Geometry: final body of the model. Coordinates: model frame, mm. Face numbers are marked on the shaded views. A direction names the side the tool comes from. Coordinates: 2 decimals unless noted, no trailing zeros. Loops run counter-clockwise (first coordinate to the right, second up) from the corner with the lowest first, then second, coordinate; pieces in that order, holes last. Notation, with made-up numbers: M 48.25,52.25 L 94.25,52.25 A16 ccw 94.25,64.25 Z; hole C -26,-14 d11. An arc over 180 degrees is marked long. Write each question's results on one line, items separated by ' | '. Start each with the question number.
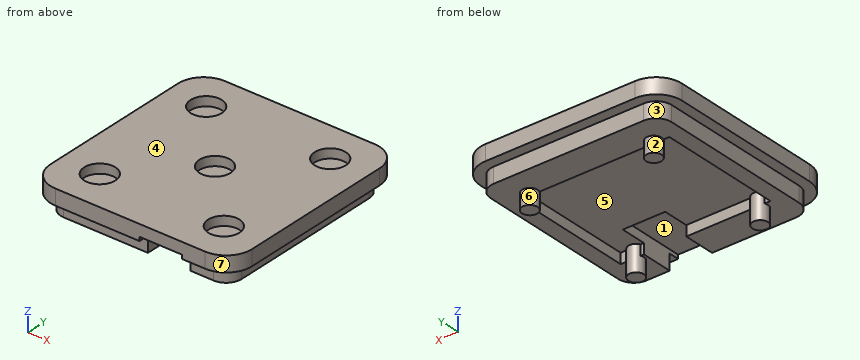
Autodesk Fusion 360 part; units mm, degrees
sketch "Outline camera" plane through (0, 0, 0) normal (0, 0, 1) x (1, 0, 0)
  line L0 (-6.5, 6.5) -> (-2.5981, 6.5)
  line L1 (2.5981, 6.5) -> (6.5, 6.5)
  arc A0 (6.7082, 2) -> (6.5, 2.5981) centre (0, 0) ccw
  arc A1 (2.5981, 6.5) -> (-2.5981, 6.5) centre (0, 0) ccw
  line L2 (6.7082, 2) -> (9, 2)
  line L3 (6.5, 6.5) -> (6.5, 2.5981)
  line L4 (6.5, -2.5981) -> (6.5, -6.5)
  arc A2 (9, -2) -> (9, 2) centre (9, 0) ccw
  line L5 (9, -2) -> (6.7082, -2)
  arc A3 (6.5, -2.5981) -> (6.7082, -2) centre (0, 0) ccw
  line L6 (6.5, -6.5) -> (2.5981, -6.5)
  line L7 (-2.5981, -6.5) -> (-6.5, -6.5)
  line L8 (-9, 2) -> (-6.7082, 2)
  line L9 (-6.7082, -2) -> (-9, -2)
  line L10 (-6.5, -6.5) -> (-6.5, -2.5981)
  line L11 (-6.5, 2.5981) -> (-6.5, 6.5)
  arc A4 (-9, 2) -> (-9, -2) centre (-9, 0) ccw
  arc A5 (-6.5, 2.5981) -> (-6.7082, 2) centre (0, 0) ccw
  arc A6 (-6.7082, -2) -> (-6.5, -2.5981) centre (0, 0) ccw
  arc A7 (-2.5981, -6.5) -> (2.5981, -6.5) centre (0, 0) ccw
  arc A8 (2.6926, 7) -> (-2.6926, 7) centre (0, 0) ccw
  line L12 (-7, 7) -> (-2.6926, 7)
  line L13 (-7, 2.6926) -> (-7, 7)
  arc A9 (-7, 2.6926) -> (-7.0711, 2.5) centre (0, 0) ccw
  line L14 (-9, 2.5) -> (-7.0711, 2.5)
  arc A10 (-9, 2.5) -> (-9, -2.5) centre (-9, 0) ccw
  line L15 (-7.0711, -2.5) -> (-9, -2.5)
  arc A11 (-7.0711, -2.5) -> (-7, -2.6926) centre (0, 0) ccw
  line L16 (-7, -7) -> (-7, -2.6926)
  line L17 (-2.6926, -7) -> (-7, -7)
  arc A12 (-2.6926, -7) -> (2.6926, -7) centre (0, 0) ccw
  line L18 (7, -7) -> (2.6926, -7)
  line L19 (7, -2.6926) -> (7, -7)
  arc A13 (7, -2.6926) -> (7.0711, -2.5) centre (0, 0) ccw
  line L20 (9, -2.5) -> (7.0711, -2.5)
  arc A14 (9, -2.5) -> (9, 2.5) centre (9, 0) ccw
  line L21 (7.0711, 2.5) -> (9, 2.5)
  arc A15 (7.0711, 2.5) -> (7, 2.6926) centre (0, 0) ccw
  line L22 (7, 7) -> (7, 2.6926)
  line L23 (2.6926, 7) -> (7, 7)
  dimension "d3" = 13
  dimension "d4" = 13
  dimension "d5" = 14
  dimension "d6" = 4
  dimension "d7" = 4
  dimension "d8" = 2
  dimension "d9" = 2
  dimension "d11" = 9
  dimension "d12" = 9
  dimension "d18" = -0.5
sketch "Box size" plane through (0, 0, 0) normal (0, 0, 1) x (1, 0, 0)
  line L0 (19.5, 20.125) -> (-19.5, 20.125)
  line L1 (-19.5, 20.125) -> (-19.5, -20.125)
  line L2 (-19.5, -20.125) -> (19.5, -20.125)
  line L3 (19.5, -20.125) -> (19.5, 20.125)
  line L4 (19.5, 20.125) -> (-19.5, -20.125) construction
  line L5 (-19.5, 20.125) -> (19.5, -20.125) construction
  line L6 (-14.5, -18.125) -> (14.5, -18.125)
  line L7 (17.5, -15.125) -> (17.5, 15.125)
  line L8 (14.5, 18.125) -> (-14.5, 18.125)
  line L9 (-17.5, 15.125) -> (-17.5, -15.125)
  arc A0 (17.5, 15.125) -> (14.5, 18.125) centre (14.5, 15.125) ccw
  arc A1 (-14.5, 18.125) -> (-17.5, 15.125) centre (-14.5, 15.125) ccw
  arc A2 (14.5, -18.125) -> (17.5, -15.125) centre (14.5, -15.125) ccw
  arc A3 (-17.5, -15.125) -> (-14.5, -18.125) centre (-14.5, -15.125) ccw
  dimension "d13" = 39
  dimension "d14" = 40.25
  dimension "d47" = 3
sketch "LEDs" plane through (0, 0, 0) normal (0, 0, 1) x (1, 0, 0)
  circle A0 centre (-12.5, 6) radius 2.4
  line L0 (0, 2.5) -> (0, 20)
  circle A1 centre (12.5, 6) radius 2.4
  line L1 (20, 0) -> (2.5, 0)
  circle A2 centre (-12.5, -6) radius 2.4
  circle A3 centre (12.5, -6) radius 2.4
  dimension "d15" = 4.8
  dimension "d16" = 12.5
  dimension "d17" = 6
extrude "Extrude1" add sketch "Box size" along normal blind 6 contours L0 L1 L2 L3 | L6 L7 L8 L9 A0 A1 A2 A3
sketch "Pins" plane through (0, 0, 0) normal (0, 0, 1) x (1, 0, 0)
  line L0 (12, 12.625) -> (-12, 12.625)
  line L1 (-12, 12.625) -> (-12, -12.625)
  line L2 (-12, -12.625) -> (12, -12.625)
  line L3 (12, -12.625) -> (12, 12.625)
  line L4 (12, 12.625) -> (-12, -12.625) construction
  line L5 (-12, 12.625) -> (12, -12.625) construction
  circle A0 centre (-12, -12.625) radius 1.5
  circle A1 centre (12, -12.625) radius 1.5
  circle A2 centre (12, 12.625) radius 1.5
  circle A3 centre (-12, 12.625) radius 1.5
  dimension "d35" = 24
  dimension "d36" = 25.25
  dimension "d37" = 3
extrude "Extrude4" add sketch "Pins" against normal blind 3 contours L0 L1 A3 | L0 L1 A3 | L0 L3 A2 | L0 L3 A2 | L1 L2 A0 | L1 L2 A0 | L2 L3 A1 | L2 L3 A1
fillet "Fillet2" radius 5 4 edges at (-19.5, 20.125, 3) (-19.5, -20.125, 3) (19.5, -20.125, 3) (19.5, 20.125, 3)
extrude "Extrude6" cut sketch "Box size" along normal blind 3
sketch "Sketch15" plane through (0, 0, 0) normal (0, 0, -1) x (1, 0, 0)
  circle A0 centre (-12, -12.625) radius 1.5
  circle A1 centre (-12, 12.625) radius 1.5
  circle A2 centre (12, -12.625) radius 1.5
  circle A3 centre (12, 12.625) radius 1.5
  arc A4 (-14.5, 18.125) -> (-17.5, 15.125) centre (-14.5, 15.125) ccw
  line L0 (-17.5, 15.125) -> (-17.5, -15.125)
  arc A5 (-17.5, -15.125) -> (-14.5, -18.125) centre (-14.5, -15.125) ccw
  line L1 (-14.5, -18.125) -> (14.5, -18.125)
  arc A6 (14.5, -18.125) -> (17.5, -15.125) centre (14.5, -15.125) ccw
  line L2 (17.5, -15.125) -> (17.5, 15.125)
  arc A7 (17.5, 15.125) -> (14.5, 18.125) centre (14.5, 15.125) ccw
  line L3 (14.5, 18.125) -> (-14.5, 18.125)
  line L4 (-14.5, 12) -> (14.5, 12)
  line L5 (14.5, 12) -> (14.5, -12)
  line L6 (14.5, -12) -> (-14.5, -12)
  line L7 (-14.5, -12) -> (-14.5, 12)
  line L8 (-14.5, 12) -> (14.5, -12) construction
  line L9 (14.5, 12) -> (-14.5, -12) construction
  dimension "d55" = 29
  dimension "d56" = 24
extrude "Extrude11" cut sketch "Sketch15" against normal blind 2 contours A0 A1 A2 A3 L4 L5 L6 L7
sketch "cable" plane through (0, 0, 0) normal (0, 0, -1) x (1, 0, 0)
  line L0 (-14.5, -12) -> (-13.3636, -12)
  arc A0 (-10.6364, -12) -> (-13.3636, -12) centre (-12, -12.625) ccw
  line L1 (-10.6364, -12) -> (10.6364, -12)
  arc A1 (13.3636, -12) -> (10.6364, -12) centre (12, -12.625) ccw
  line L2 (13.3636, -12) -> (14.5, -12)
  line L3 (14.5, -12) -> (14.5, 12)
  line L4 (14.5, 12) -> (13.3636, 12)
  arc A2 (10.6364, 12) -> (13.3636, 12) centre (12, 12.625) ccw
  line L5 (10.6364, 12) -> (-10.6364, 12)
  arc A3 (-13.3636, 12) -> (-10.6364, 12) centre (-12, 12.625) ccw
  line L6 (-13.3636, 12) -> (-14.5, 12)
  line L7 (-14.5, 12) -> (-14.5, -12)
  line L8 (10, 7) -> (1.8, 7)
  line L9 (1.8, 7) -> (1.8, 27)
  line L10 (1.8, 27) -> (10, 27)
  line L11 (10, 27) -> (10, 7)
  line L12 (14.5, 18.125) -> (-14.5, 18.125)
  arc A4 (-14.5, 18.125) -> (-17.5, 15.125) centre (-14.5, 15.125) ccw
  line L13 (-17.5, 15.125) -> (-17.5, -15.125)
  arc A5 (-17.5, -15.125) -> (-14.5, -18.125) centre (-14.5, -15.125) ccw
  line L14 (-14.5, -18.125) -> (14.5, -18.125)
  arc A6 (14.5, -18.125) -> (17.5, -15.125) centre (14.5, -15.125) ccw
  line L15 (17.5, -15.125) -> (17.5, 15.125)
  arc A7 (17.5, 15.125) -> (14.5, 18.125) centre (14.5, 15.125) ccw
  line L16 (13.3636, 12) -> (14.5, 12)
  line L17 (14.5, 12) -> (14.5, -12)
  line L18 (14.5, -12) -> (13.3636, -12)
  arc A8 (10.6364, -12) -> (13.3636, -12) centre (12, -12.625) ccw
  line L19 (10.6364, -12) -> (-10.6364, -12)
  arc A9 (-13.3636, -12) -> (-10.6364, -12) centre (-12, -12.625) ccw
  line L20 (-13.3636, -12) -> (-14.5, -12)
  line L21 (-14.5, -12) -> (-14.5, 12)
  line L22 (-14.5, 12) -> (-13.3636, 12)
  arc A10 (-10.6364, 12) -> (-13.3636, 12) centre (-12, 12.625) ccw
  line L23 (-10.6364, 12) -> (10.6364, 12)
  arc A11 (13.3636, 12) -> (10.6364, 12) centre (12, 12.625) ccw
  dimension "d67" = 8.2
  dimension "d68" = 2
  dimension "d69" = 20
extrude "Extrude12" cut sketch "cable" against normal blind 3.75 contours L5 L9 L11 L12 L23 | L5 L8 L9 L11 L23 | L9 L10 L11 L12
sketch "Sketch17" plane through (0, 0, 6) normal (0, 0, 1) x (-1, 0, 0)
  arc A0 (-19.5, -15.125) -> (-14.5, -20.125) centre (-14.5, -15.125) ccw
  line L0 (-14.5, -20.125) -> (14.5, -20.125)
  arc A1 (14.5, -20.125) -> (19.5, -15.125) centre (14.5, -15.125) ccw
  line L1 (19.5, -15.125) -> (19.5, 15.125)
  arc A2 (19.5, 15.125) -> (14.5, 20.125) centre (14.5, 15.125) ccw
  line L2 (14.5, 20.125) -> (-14.5, 20.125)
  arc A3 (-14.5, 20.125) -> (-19.5, 15.125) centre (-14.5, 15.125) ccw
  line L3 (-19.5, 15.125) -> (-19.5, -15.125)
  circle A4 centre (-12, 12.625) radius 3.025
  circle A5 centre (0, 0) radius 3.025
  dimension "d72" = 6.05
  dimension "d75" = 7.5
  dimension "d76" = 7.5
extrude "Extrude13" cut sketch "Sketch17" against normal blind 1.8 contours A4 | A5
mirror "Mirror1" about plane through (0, 0, 0) normal (0, 1, 0) of "Extrude13"
mirror "Mirror2" about plane through (0, 0, 0) normal (1, 0, 0) of "Extrude13", "Mirror1"
equation "d13 = 34 mm + 5 mm"
equation "d14 = 32 mm + 4 mm - 1 mm + 0.25 mm + 5 mm"
equation "d36 = 22 mm + 4 mm - 1 mm + 0.25 mm"
Item 1: Section A-A, the plane y = 0. Return loops of the section in (x, z) (3 decimals).
Item 2: Pull-direction query (Y, two-part tool) for the marked faces 4, 5, 6 and 7; classes: released by +Y, released by -Y, zero draft, split by the parting line, or undercut.
Item 3: Section D-D, the plane x = 0. Return loops of the section in (y, z) (3 decimals).
Item 4: Contact query for flat-ended pins moving along their axis: P1, Ø1, axis at x = 1, z = 1.5, coming from the -Y side (3 decimals); P2, Ø3, axis at x = -10.5, y = -2.5, coming from the -Z side; P3, Ø0.9, axis at x = 6, z = 1, coming from the +Y side (3 decimals). Output: stop coordinate, or through.
Item 5: Section C-C, the plane z = 0.5. Return loops of the section in (x, y) (3 decimals), plus the area to 3 significant figures.
Item 6: Section B-B, the plane x = -12. Return loops of the section in (y, z) (3 decimals), plus the area to 3 significant figures.
Item 7: Set-up query: the marked faces 1, 2 and 3. Return all of +Z, -Z, +X, -X, +Y, -Y with unobstructed straight access to the full face (end or side cutting, diameter ignored); none if empty.
Item 8: Ray query, L1, parallel to Y at x = -12, z = 4.95 (3 decimals); L2, parallel to X at y = 10, z = 4.25; L3, parallel to Y at x = 0, z = 4.9 (3 decimals). Return the intervals inside material, ascending. Write a range as [from, to].
Solutions:
1) outline: M -19.5,3 L -17.5,3 L -17.5,0 L -14.5,0 L -14.5,2 L 14.5,2 L 14.5,0 L 17.5,0 L 17.5,3 L 19.5,3 L 19.5,6 L 3.025,6 L 3.025,4.2 L -3.025,4.2 L -3.025,6 L -19.5,6 Z
2) face 4: zero draft | face 5: undercut | face 6: undercut | face 7: released by -Y
3) outline: M -20.125,3 L -18.125,3 L -18.125,0 L -12,0 L -12,2 L 12,2 L 12,0 L 18.125,0 L 18.125,3 L 20.125,3 L 20.125,6 L 3.025,6 L 3.025,4.2 L -3.025,4.2 L -3.025,6 L -20.125,6 Z
4) P1: stops at y = -18.125 | P2: stops at z = 2 | P3: stops at y = 18.125
5) outline: M -17.5,-15.125 A3 ccw -14.5,-18.125 L 1.8,-18.125 L 1.8,-12 L -10.636,-12 A1.5 ccw -13.364,-12 L -14.5,-12 L -14.5,12 L -13.364,12 A1.5 ccw -10.636,12 L 10.636,12 A1.5 ccw 13.364,12 L 14.5,12 L 14.5,-12 L 13.364,-12 A1.5 ccw 10.636,-12 L 10,-12 L 10,-18.125 L 14.5,-18.125 A3 ccw 17.5,-15.125 L 17.5,15.125 A3 ccw 14.5,18.125 L -14.5,18.125 A3 ccw -17.5,15.125 Z | area: 522 mm²
6) outline: M -20.125,3 L -18.125,3 L -18.125,0 L -14.125,0 L -14.125,-3 L -11.125,-3 L -11.125,2 L 11.125,2 L 11.125,-3 L 14.125,-3 L 14.125,0 L 18.125,0 L 18.125,3 L 20.125,3 L 20.125,6 L 15.65,6 L 15.65,4.2 L 9.6,4.2 L 9.6,6 L -9.6,6 L -9.6,4.2 L -15.65,4.2 L -15.65,6 L -20.125,6 Z | area: 181 mm²
7) face 1: -Z, -Y | face 2: -Z | face 3: -Z, -X, +Y
8) L1: y = [-20.125, -15.65], [-9.6, 9.6], [15.65, 20.125] | L2: x = [-19.5, -13.5], [-10.5, 10.5], [13.5, 19.5] | L3: y = [-20.125, -3.025], [3.025, 20.125]
